Read the model definition and answer for the solid it produces. Units are mm, in the model's axes. Coordinates: 2 decimals unless noted, no trailing zeros. Loops run counter-clockwise (first coordinate to the right, second up) from the corner with the lowest first, then second, coordinate; pieces in that order, holes last. Notation, with made-up numbers: (-8.75, -8.75) - (0.25, -8.75) arc R17 ccw to (0.25, 3.25) - close; hole circle Ø6 at (33.25, 62.5). An arc over 180 degrees is marked (long way). Use CSV: the item, a comma, the result in double quotes.
Autodesk Inventor part; units mm, degrees
ref_plane "YZ Plane" through (0, 0, 0) normal (1, 0, 0) x (0, 1, 0)
ref_plane "XZ Plane" through (0, 0, 0) normal (0, 1, 0) x (-1, 0, 0)
ref_plane "XY Plane" through (0, 0, 0) normal (0, 0, 1) x (1, 0, 0)
sketch "Sketch1" plane through (0, 0, 0) normal (0, 1, 0) x (-1, 0, 0)
  line L0 (10, -45) -> (-10, -45)
  line L1 (-10, -45) -> (-10, 45)
  line L2 (-10, 45) -> (10, 45)
  line L3 (10, 45) -> (10, -45)
  point P0 (0, 0)
  dimension "d0" = 20
  dimension "d1" = 90
  dimension "d2" = 45
  dimension "d3" = 10
extrude "Plate1" add sketch "Sketch1" along normal blind 1.5
sketch "Sketch2" plane through (0, 0, 0) normal (0, -1, 0) x (1, 0, 0)
  circle A0 centre (0, 42) radius 0.7835
  circle A1 centre (-7, 35) radius 0.7835
  circle A2 centre (0, 28) radius 0.7835
  circle A3 centre (7, 35) radius 0.7835
  circle A4 centre (0, -28) radius 0.7835
  circle A5 centre (-7, -35) radius 0.7835
  circle A6 centre (0, -42) radius 0.7835
  circle A7 centre (7, -35) radius 0.7835
  point P0 (0, 0)
hole "Hole1" at (0, 0, 42) at (-7, 0, 35) at (0, 0, 28) at (7, 0, 35) at (0, 0, -28) at (-7, 0, -35) at (0, 0, -42) at (7, 0, -35) direction (0, 1, 0) diameter 2.1 depth 1.5
sketch "Sketch3" plane through (0, 1.5, 0) normal (0, 1, 0) x (1, 0, 0)
  arc A0 (10, 35) -> (-10, 35) centre (0, 35) ccw
  arc A1 (-10, -35) -> (10, -35) centre (0, -35) ccw
  line L0 (-10, 35) -> (-10, -35)
  line L1 (10, 35) -> (10, -35)
  line L2 (10, 45) -> (10, -45)
  line L3 (-10, 45) -> (10, 45)
  line L4 (10, 45) -> (10, -45)
  line L5 (10, -45) -> (-10, -45)
  line L6 (-10, -45) -> (-10, 45)
  point P0 (0, 0)
  point P1 (0, 45)
  point P2 (10, 35)
  point P3 (-10, -35)
  point P4 (0, -45)
  point P5 (10, -35)
  dimension "d12" = 35
  dimension "d13" = 35
  dimension "d14" = 10
  dimension "d15" = 10
  dimension "d16" = 10
  dimension "d17" = 20
  dimension "d18" = 90
extrude "Extrusion1" cut sketch "Sketch3" against normal blind 10 contours A0 L3 L2 | A0 L6 L3 | L2 L5 A1 | L5 L6 A1
sketch "Sketch4" plane through (0, 0, 0) normal (0, -1, 0) x (1, 0, 0)
  arc A0 (-10, -35) -> (10, -35) centre (0, -35) ccw
  arc A1 (10, 35) -> (-10, 35) centre (0, 35) ccw
  point P0 (0, 0)
hole "Hole2" at (0, 0, 35) at (0, 0, -35) direction (0, 1, 0) diameter 7.2 depth 1.5
equation "\"d10\" = Thickness"
equation "\"d26\" = Thickness"
equation "\"d4\" = Thickness"
equation "\"BendReliefWidth\" = Thickness"
equation "\"BendReliefDepth\" = 0.5 * Thickness"
equation "\"CornerReliefSize\" = 4 * Thickness"
equation "\"MinimumRemnant\" = 2 * Thickness"
equation "\"TransitionRadius\" = BendRadius"
equation "\"JacobiRadiusSize\" = BendRadius"
equation "\"GapSize\" = Thickness"
properties part number "axis_10_11-connector_frame" material "Aluminum 6061-AHC"
Q1. The part is cut by section C-C on y = 0.3. Give the number of separate pieces and of enclosed holes in the cut face, and give its area (3 significant figures).
Reported:
separate pieces,"1"
enclosed holes,"10"
area,"1,610 mm²"
Q2. The part is cut by section B-B on x = 0. Determine the outline of the cut face in (y, z), and give its area (3 significant figures).
Reported:
outline,"(0, -45) - (1.5, -45) - (1.5, -43.05) - (0, -43.05) - close; (0, -40.95) - (1.5, -40.95) - (1.5, -38.6) - (0, -38.6) - close; (0, -31.4) - (1.5, -31.4) - (1.5, -29.05) - (0, -29.05) - close; (0, -26.95) - (1.5, -26.95) - (1.5, 26.95) - (0, 26.95) - close; (0, 29.05) - (1.5, 29.05) - (1.5, 31.4) - (0, 31.4) - close; (0, 38.6) - (1.5, 38.6) - (1.5, 40.95) - (0, 40.95) - close; (0, 43.05) - (1.5, 43.05) - (1.5, 45) - (0, 45) - close"
area,"101 mm²"
Q3. The part is cut by section A-A on z = -28. Determine the outline of the cut face in (x, y), and give its area (4 significant figures).
Reported:
outline,"(-10, 0) - (-1.05, 0) - (-1.05, 1.5) - (-10, 1.5) - close; (1.05, 0) - (10, 0) - (10, 1.5) - (1.05, 1.5) - close"
area,"26.85 mm²"
Q4. The part is cut by section D-D on x = -7. Determine the outline of the cut face in (y, z).
Reported:
outline,"(0, -42.14) - (1.5, -42.14) - (1.5, -36.05) - (0, -36.05) - close; (0, -33.95) - (1.5, -33.95) - (1.5, 33.95) - (0, 33.95) - close; (0, 36.05) - (1.5, 36.05) - (1.5, 42.14) - (0, 42.14) - close"
Q5. Find the intervals of material crossed by probe 1 along X at (y, z) = (0.5, -35); probe 2 along X at (y, z) = (1.05, 28); probe 3 along Z at (x, y) = (7, 0.35), in increasing order. Write a range as [from, to].
Reported:
probe 1,"x = [-10, -8.05], [-5.95, -3.6], [3.6, 5.95], [8.05, 10]"
probe 2,"x = [-10, -1.05], [1.05, 10]"
probe 3,"z = [-42.14, -36.05], [-33.95, 33.95], [36.05, 42.14]"
Q6. For a pull along Z with two mould halves and no side action, classify faces 1 (the face through (0, 1, 45)), 2 (the face through (0, 1, -45)), 3 (the face through (-0.05, 0.76, -40.95)) as +Z half, -Z half, draft (parallel to the pull), parting line (faces both ways), or undercut.
Reported:
face 1,"+Z half"
face 2,"-Z half"
face 3,"undercut"
